Part print with two shaded views. Sizes in mm from the minimum x, y, z corner. Round coordinates to 2 decimals unless told otherwise and drop trailing zeros. Write each loop counter-clockwise with the first axis right and the second up, starting at its lowest first coordinate (ties: lowest second). Pieces come first, ordered by that corner, then holes. Notation, with made-up numbers: (58, 15.5) - (96, 15.5) arc R13 ccw to (96, 27.5) - close; hole circle Ø6 at (74.25, 89.25). An arc over 180 degrees is marked (long way). Answer as a JSON object with one key per item and string values. Group by question number.
Item 1: Slice it at A-A, the plane x = 65. List the corners of the cut face in (y, z).
Item 2: Flat gauge pins, fed straight in: pin 1 (3 mm diameter, centred on x = 71.5, y = 1.5, fed in from -Z); pin 2 (3 mm diameter, centred on y = 3, z = 62, fed in from -X); pin 3 (3 mm diameter, centred on x = 57.5, y = 4, fed in from +Z). Where does each tip first touch, or does it go through?
Item 3: Probe line 1 (Z direction, x = 119.5, y = 3.4); line 2 (X direction, y = 1.45, z = 62); line 3 (X direction, y = 3.5, z = 139). List the from-to ranges inside material, lowest first. Write a range as from..to.
Item 4: Slice it at D-D, the plane y = 5. Give the number of separate pieces and of enclosed holes in the cut face, then the cut area to 3 significant figures.
Item 5: Slice it at B-B, the plane z = 56. List the corners of the cut face in (x, y).
Item 6: Slice it at C-C, the plane z = 139. List the corners of the cut face in (x, y), then the cut area to 3 significant figures.
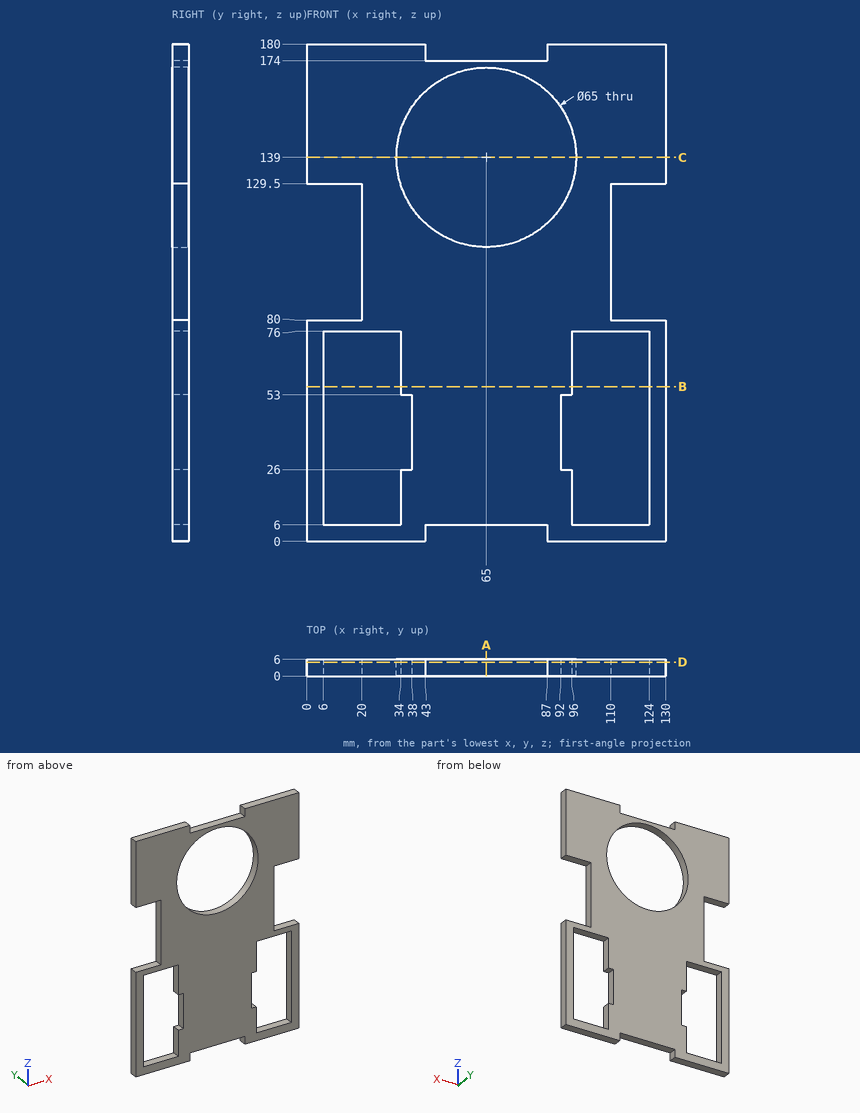
Geometry says:
{
 "1": {"outline": "(0, 6) - (6, 6) - (6, 106.5) - (0, 106.5) - close; (0, 171.5) - (6, 171.5) - (6, 174) - (0, 174) - close"},
 "2": {"pin 1": "stops at z = 6", "pin 2": "stops at x = 0", "pin 3": "stops at z = 174"},
 "3": {"line 1": "z = 0..6, 76..80, 129.5..180", "line 2": "x = 0..6, 34..96, 124..130", "line 3": "x = 0..32.5, 97.5..130"},
 "4": {"separate pieces": "1", "enclosed holes": "3", "area": "13,400 mm^2"},
 "5": {"outline": "(0, 0) - (6, 0) - (6, 6) - (0, 6) - close; (34, 0) - (96, 0) - (96, 6) - (34, 6) - close; (124, 0) - (130, 0) - (130, 6) - (124, 6) - close"},
 "6": {"outline": "(0, 0) - (32.5, 0) - (32.5, 6) - (0, 6) - close; (97.5, 0) - (130, 0) - (130, 6) - (97.5, 6) - close", "area": "390 mm^2"}
}
